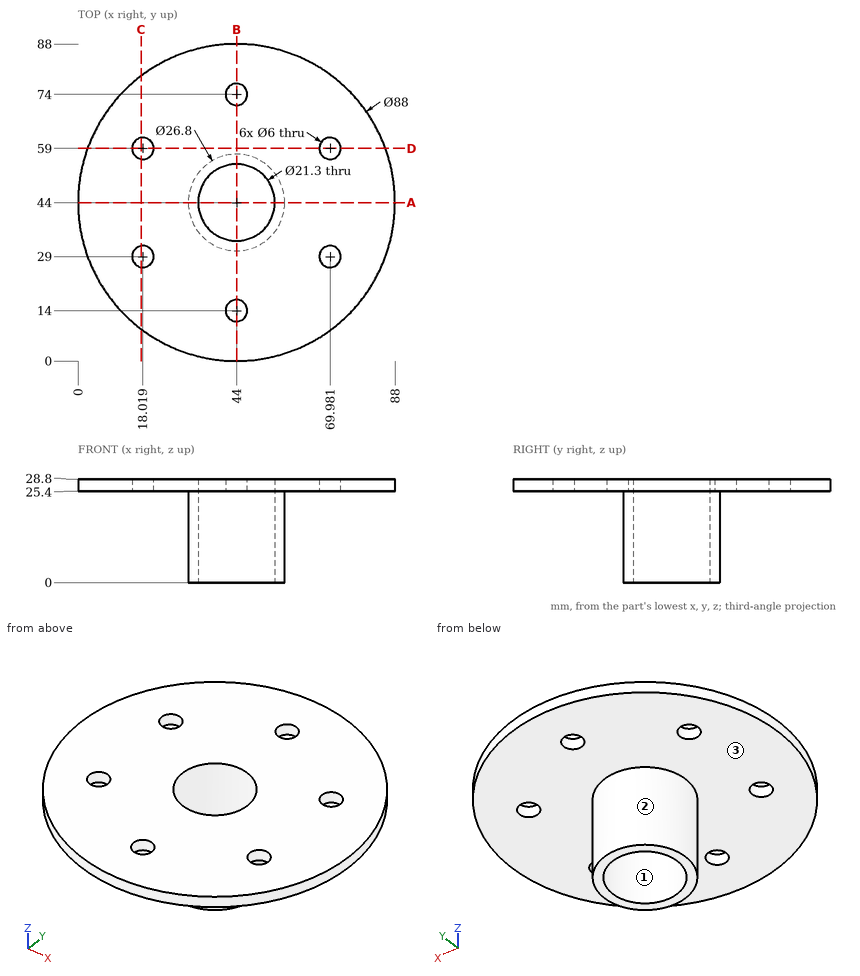
Drawing for the job (mm, zero at the part's lowest x, y, z). Give positions to 0.01 mm unless a question says otherwise; leave off trailing zeros. Loops run counter-clockwise (first coordinate to the right, second up) from the corner with the lowest first, then second, coordinate; pieces in that order, holes last. Notation, with made-up numbers: M 24.5,43.5 L 28.5,43.5 A16 cw 28.5,64.5 Z; hole C 72,53 d8. An arc over 180 degrees is marked long. One line per question, with ' | ' between items. Start each with the question number.
1. Two-plate mould, pull along X, no slides. Class the marked faces 1, 2 and 3: pulls with the +X half, pulls with the -X half, needs draft (parallel to the pull), parting line crosses it, or undercut.
2. Saw through at C-C on x = 17.5. Give the cut face in (y, z) (1 decimal).
3. Flat gauge pins, fed straight in: pin 1 (3 mm diameter, centred on x = 41, z = 7.5, fed in from +Y); pin 2 (12 mm diameter, centred on y = 50.5, z = 9.5, fed in from +X); pin 3 (5 mm diameter, centred on x = 44, y = 74, fed in from -Z); pin 4 (1 mm diameter, centred on y = 35.5, z = 23.5, fed in from +X). Where does each tip first touch, or does it go through?
4. Probe L1, parallel to Y at x = 44, z = 26.4; L2, parallel to Y at x = 43, z = 26.25; L3, parallel to Z at x = 75.5, y = 61. List the from-to ranges inside material, lowest first. Write a range as from..to.
5. Saw through at B-B on x = 44. Give the cut face in (y, z), plus the area to 3 significant figures.
6. Saw through at A-A on y = 44. Give the cut face in (x, z).
7. Saw through at D-D on y = 59. Give the cut face in (x, z).
Result sheet:
1) face 1: undercut | face 2: parting line crosses it | face 3: needs draft
2) outline: M 8.9,25.4 L 26,25.4 L 26,28.8 L 8.9,28.8 Z; M 32,25.4 L 56,25.4 L 56,28.8 L 32,28.8 Z; M 62,25.4 L 79.1,25.4 L 79.1,28.8 L 62,28.8 Z
3) pin 1: stops at y = 57.32 | pin 2: stops at x = 57.39 | pin 3: passes through | pin 4: stops at x = 54.75
4) L1: y = 0..11, 17..33.35, 54.65..71, 77..88 | L2: y = 0.01..11.17, 16.83..33.4, 54.6..71.17, 76.83..87.99 | L3: z = 25.4..28.8
5) outline: M 0,25.4 L 11,25.4 L 11,28.8 L 0,28.8 Z; M 17,25.4 L 30.6,25.4 L 30.6,0 L 33.35,0 L 33.35,28.8 L 17,28.8 Z; M 54.65,0 L 57.4,0 L 57.4,25.4 L 71,25.4 L 71,28.8 L 54.65,28.8 Z; M 77,25.4 L 88,25.4 L 88,28.8 L 77,28.8 Z | area: 326 mm^2
6) outline: M 0,25.4 L 30.6,25.4 L 30.6,0 L 33.35,0 L 33.35,28.8 L 0,28.8 Z; M 54.65,0 L 57.4,0 L 57.4,25.4 L 88,25.4 L 88,28.8 L 54.65,28.8 Z
7) outline: M 2.64,25.4 L 15.02,25.4 L 15.02,28.8 L 2.64,28.8 Z; M 21.02,25.4 L 66.98,25.4 L 66.98,28.8 L 21.02,28.8 Z; M 72.98,25.4 L 85.36,25.4 L 85.36,28.8 L 72.98,28.8 Z
